The model under review builds one solid part; all positions refer to its coordinate system, in mm. Coordinates: 2 decimals unless noted, no trailing zeros. Write each loop counter-clockwise with the first axis right and the second up, starting at its lowest first coordinate (ties: lowest second). Pieces come first, ordered by that corner, then holes.
```python
from build123d import *

# Parameters (mm, degrees)
SKETCH_W        = 73
SKETCH_H        = 48
PAD_DEPTH       = 2
FILLET_R        = 1
FILLET001_R     = 1
FILLET002_R     = 1
FILLET003_R     = 1
SKETCH002_R     = 1.5
POCKET_DEPTH    = 5
SKETCH003_R     = 1.5
POCKET001_DEPTH = 5
SKETCH004_R     = 1.5
POCKET002_DEPTH = 5
SKETCH005_R     = 1.5
POCKET003_DEPTH = 5
CHAMFER_SIZE    = 1
CHAMFER001_SIZE = 1
CHAMFER002_SIZE = 1
CHAMFER003_SIZE = 1


with BuildPart() as part:
    # Sketch → Pad (new body)
    with BuildSketch(Plane.XY):
        with Locations((36.5, 24)):
            Rectangle(SKETCH_W, SKETCH_H)
    extrude(amount=PAD_DEPTH)

    # Fillet
    fillet_edges = [part.edges().sort_by_distance(p)[0] for p in [
        (0, 0, 1),
    ]]
    fillet(fillet_edges, radius=FILLET_R)

    # Fillet001
    fillet001_edges = [part.edges().sort_by_distance(p)[0] for p in [
        (73, 0, 1),
    ]]
    fillet(fillet001_edges, radius=FILLET001_R)

    # Fillet002
    fillet002_edges = [part.edges().sort_by_distance(p)[0] for p in [
        (73, 48, 1),
    ]]
    fillet(fillet002_edges, radius=FILLET002_R)

    # Fillet003
    fillet003_edges = [part.edges().sort_by_distance(p)[0] for p in [
        (0, 48, 1),
    ]]
    fillet(fillet003_edges, radius=FILLET003_R)

    # Sketch002 (on Face10 of Fillet003) → Pocket (cut)
    with BuildSketch(Plane.XY.offset(2)):
        with Locations((3.5, 3.5)):
            Circle(SKETCH002_R)
    extrude(amount=-POCKET_DEPTH, mode=Mode.SUBTRACT)

    # Sketch003 (on Face11 of Pocket) → Pocket001 (cut)
    with BuildSketch(Plane.XY.offset(2)):
        with Locations((3.5, 44.5)):
            Circle(SKETCH003_R)
    extrude(amount=-POCKET001_DEPTH, mode=Mode.SUBTRACT)

    # Sketch004 (on Face12 of Pocket001) → Pocket002 (cut)
    with BuildSketch(Plane.XY.offset(2)):
        with Locations((69.5, 44.5)):
            Circle(SKETCH004_R)
    extrude(amount=-POCKET002_DEPTH, mode=Mode.SUBTRACT)

    # Sketch005 (on Face13 of Pocket002) → Pocket003 (cut)
    with BuildSketch(Plane.XY.offset(2)):
        with Locations((69.5, 3.5)):
            Circle(SKETCH005_R)
    extrude(amount=-POCKET003_DEPTH, mode=Mode.SUBTRACT)

    # Chamfer
    chamfer_edges = [part.edges().sort_by_distance(p)[0] for p in [
        (68, 3.5, 2),
    ]]
    chamfer(chamfer_edges, length=CHAMFER_SIZE)

    # Chamfer001
    chamfer001_edges = [part.edges().sort_by_distance(p)[0] for p in [
        (2, 44.5, 2),
    ]]
    chamfer(chamfer001_edges, length=CHAMFER001_SIZE)

    # Chamfer002
    chamfer002_edges = [part.edges().sort_by_distance(p)[0] for p in [
        (68, 44.5, 2),
    ]]
    chamfer(chamfer002_edges, length=CHAMFER002_SIZE)

    # Chamfer003
    chamfer003_edges = [part.edges().sort_by_distance(p)[0] for p in [
        (2, 3.5, 2),
    ]]
    chamfer(chamfer003_edges, length=CHAMFER003_SIZE)


solid = part.part
```
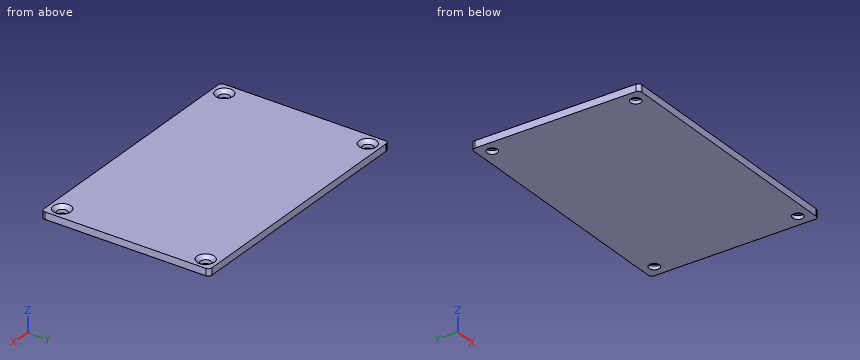
Item 1: Take a section at B-B, the plane y = 44.5. Write out the cut boundary in (x, z).
Solved:
outline: (0, 0) - (2, 0) - (2, 1) - (1, 2) - (0, 2) - close; (5, 0) - (68, 0) - (68, 1) - (67, 2) - (6, 2) - (5, 1) - close; (71, 0) - (73, 0) - (73, 2) - (72, 2) - (71, 1) - close
Item 2: Take a section at A-A, the plane x = 69.5. Write out the cut boundary in (y, z).
Solved:
outline: (0, 0) - (2, 0) - (2, 1) - (1, 2) - (0, 2) - close; (5, 0) - (43, 0) - (43, 1) - (42, 2) - (6, 2) - (5, 1) - close; (46, 0) - (48, 0) - (48, 2) - (47, 2) - (46, 1) - close
Item 3: To check wall thickness, follow line 1 along Y through (x, z) = (69.5, 0.5); line 2 along X through (y, z) = (43, 1.45); line 3 along X through (y, z) = (3, 0.15). State the ranges of each line that lie inside material, in increasing order.
Solved:
line 1: y = 0 to 2, 5 to 43, 46 to 48
line 2: x = 0 to 2.25, 4.75 to 68.25, 70.75 to 73
line 3: x = 0 to 2.09, 4.91 to 68.09, 70.91 to 73
Item 4: For pin 1 (3.5 mm diameter, centred on x = 69.5, y = 3.5, fed in from +Z); pin 2 (5 mm diameter, centred on x = 3.5, y = 3.5, fed in from -Z), all flat-tipped, find the tip position at first contact; note any pin that passes through.
Solved:
pin 1: stops at z = 1.25
pin 2: stops at z = 0
